Design review of the part shown in the three views and the two pictorial views. Dimensions are in mm from the part's minimum x, y and z. Round coordinates to 2 decimals unless told otherwise and drop trailing zeros. Order: outer loops, then holes, each group sorted by start corner. A loop starts at its lowest first (then second) coordinate and runs counter-clockwise, first axis right, second up.
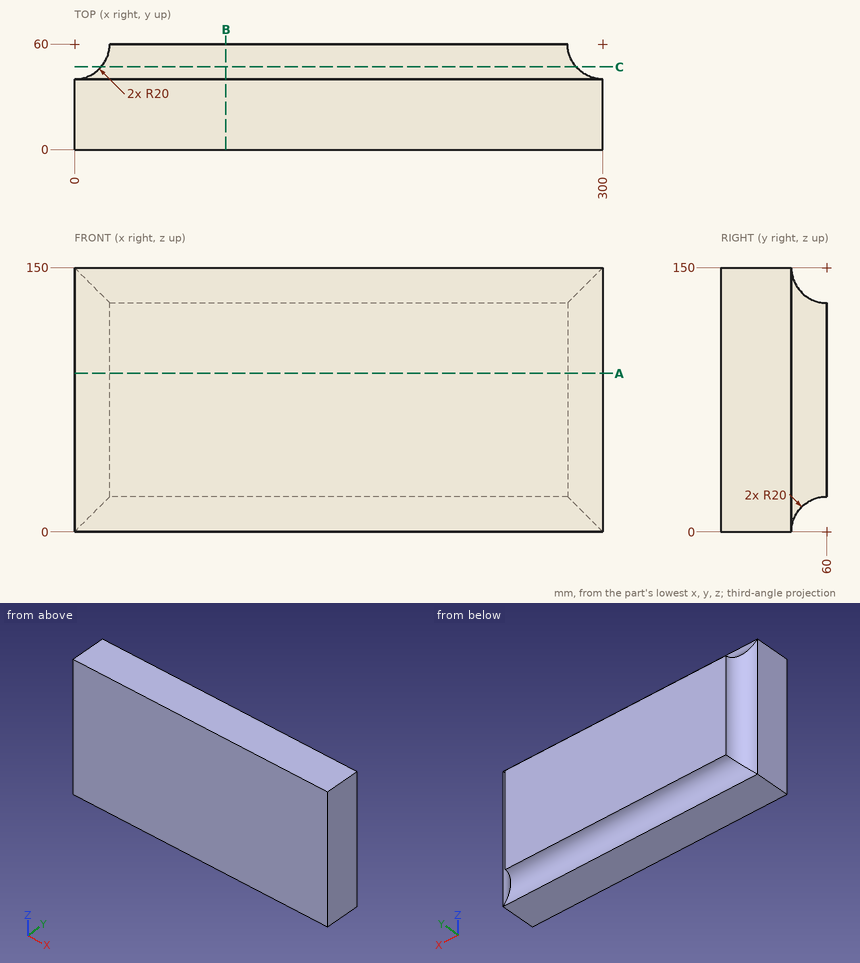
(1) Insertion check: pin 1 (1 mm diameter, centred on y = 52.5, z = 123.5, fed in from +X); pin 2 (2 mm diameter, centred on x = 49.5, y = 49.5, fed in from +Z); pin 3 (4 mm diameter, centred on x = 163.5, y = 49, fed in from -Z). Each pin has a flat end and moves straight along its axis. Give the tip position at first contact, or say it passes through.
Data:
pin 1: stops at x = 281.67
pin 2: stops at z = 133.64
pin 3: stops at z = 15.2
(2) To check wall thickness, follow probe 1 along X at (y, z) = (55, 85); probe 2 along X at (y, z) = (44, 99); probe 3 along Z at (x, y) = (90, 47). State the ranges of each line that lie inside material, in increasing order.
Data:
probe 1: x = 19.36 to 280.64
probe 2: x = 12 to 288
probe 3: z = 15.2 to 134.8
(3) Consider section C-C (y = 47). Write out the cut boundary in (x, z), and give its area (3 significant figures).
Data:
outline: (15.2, 15.2) - (284.8, 15.2) - (284.8, 134.8) - (15.2, 134.8) - close
area: 32,200 mm2
(4) Consider section B-B (x = 86). Write out the cut boundary in (y, z), and give its area (3 significant figures).
Data:
outline: (0, 0) - (40, 0) arc R20 cw to (60, 20) - (60, 130) arc R20 cw to (40, 150) - (0, 150) - close
area: 8,370 mm2
(5) Consider section A-A (z = 90). Write out the cut boundary in (x, y).
Data:
outline: (0, 0) - (300, 0) - (300, 40) arc R20 cw to (280, 60) - (20, 60) arc R20 cw to (0, 40) - close
